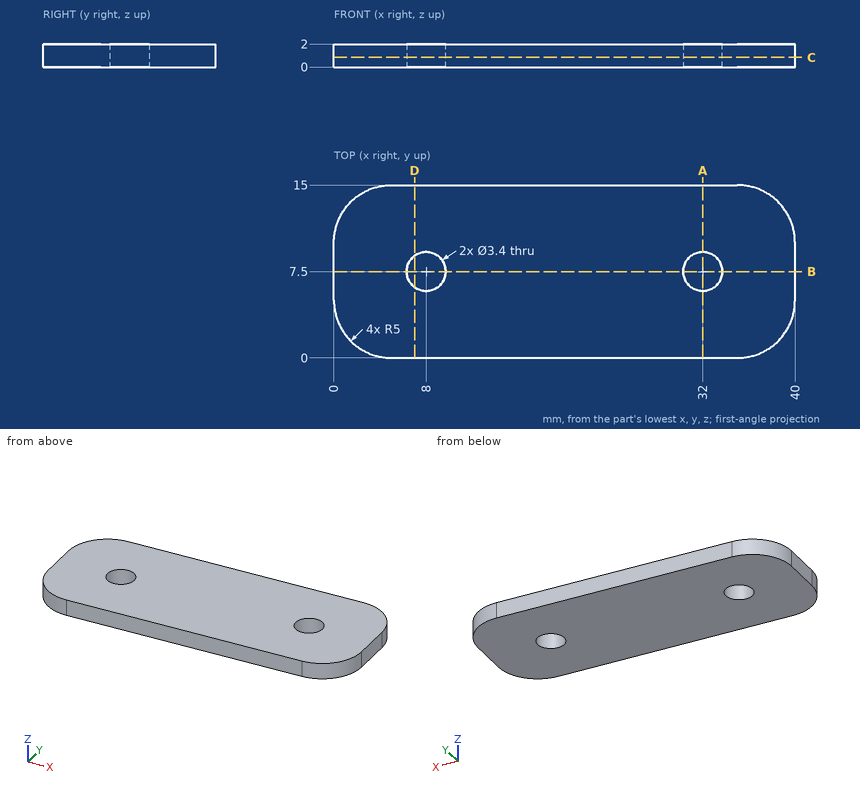
The figure shows three views and two pictorial views of one solid part (mm, origin at its lowest corner). Answer the questions. Coordinates: 2 decimals unless noted, no trailing zeros. Order: outer loops, then holes, each group sorted by start corner. A loop starts at its lowest first (then second) coordinate and runs counter-clockwise, first axis right, second up.
Q1. A cutting plane is placed at D-D, the plane x = 7. Write down the section's boundary in (y, z), and give its area (3 significant figures).
Q2. A cutting plane is placed at B-B, the plane y = 7.5. Write down the section's boundary in (x, z).
Q3. Consider line 1 (X direction, y = 7.5, z = 0.65); line 2 (Y direction, x = 8, z = 0.6); line 3 (X direction, y = 9, z = 0.4). Determine where each line is inside the solid, lowest interval first.
Q4. A cutting plane is placed at C-C, the plane z = 0.85. Write down the section's boundary in (x, y), and give its area (3 significant figures).
Q5. A cutting plane is placed at A-A, the plane x = 32. Write down the section's boundary in (y, z).
Answers follow:
1. outline: (0, 0) - (6.13, 0) - (6.13, 2) - (0, 2) - close; (8.87, 0) - (15, 0) - (15, 2) - (8.87, 2) - close
1. area: 24.5 mm2
2. outline: (0, 0) - (6.3, 0) - (6.3, 2) - (0, 2) - close; (9.7, 0) - (30.3, 0) - (30.3, 2) - (9.7, 2) - close; (33.7, 0) - (40, 0) - (40, 2) - (33.7, 2) - close
3. line 1: x = 0 to 6.3, 9.7 to 30.3, 33.7 to 40
3. line 2: y = 0 to 5.8, 9.2 to 15
3. line 3: x = 0 to 7.2, 8.8 to 31.2, 32.8 to 40
4. outline: (0, 5) arc R5 ccw to (5, 0) - (35, 0) arc R5 ccw to (40, 5) - (40, 10) arc R5 ccw to (35, 15) - (5, 15) arc R5 ccw to (0, 10) - close; hole circle Ø3.4 at (8, 7.5); hole circle Ø3.4 at (32, 7.5)
4. area: 560 mm2
5. outline: (0, 0) - (5.8, 0) - (5.8, 2) - (0, 2) - close; (9.2, 0) - (15, 0) - (15, 2) - (9.2, 2) - close
